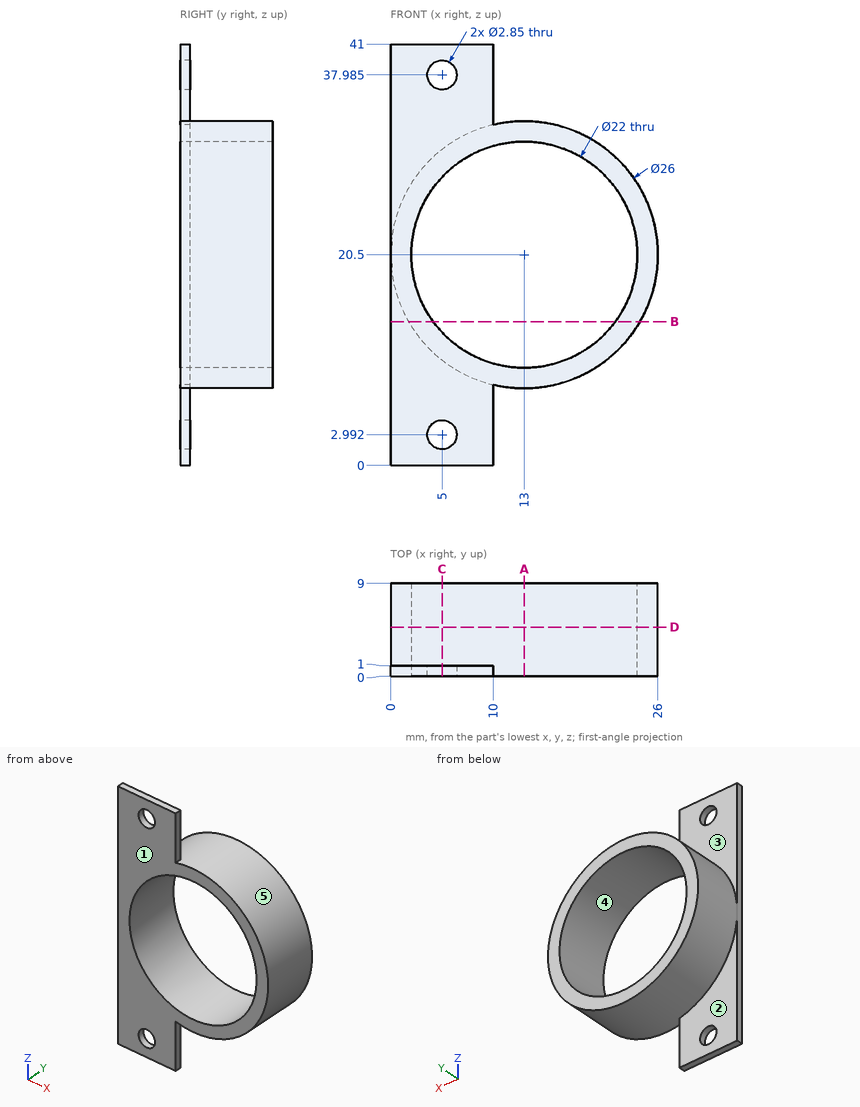
Design review of the part shown in the three views and the two pictorial views. Dimensions are in mm from the part's minimum x, y and z. A direction names the side the tool comes from. Round coordinates to 2 decimals unless told otherwise and drop trailing zeros. Write each loop counter-clockwise with the first axis right and the second up, starting at its lowest first coordinate (ties: lowest second). Pieces come first, ordered by that corner, then holes. Notation, with made-up numbers: M 18.25,38.5 L 76.25,38.5 A18 ccw 76.25,70.5 Z; hole C -21.75,-27 d4. An arc over 180 degrees is marked long. One line per item, written item: value. Start each with the question number.
1. Take a section at A-A on x = 13. State the section outline as (y, z) points.
2. Clearance check with flat-ended pins moving along their axes: P1, Ø1.1, axis at y = 0.5, z = 38, coming from the +X side; P2, Ø1, axis at y = 2, z = 10, coming from the -X side (1 decimal); P3, Ø4.5, axis at x = 5, z = 37.99, coming from the +Y side; P4, Ø13, axis at x = 13, z = 20.5, coming from the +Y side. State where each tip first meets the part, or that it passes through.
3. Take a section at B-B on z = 14. State the section outline as (x, y) points.
4. Take a section at D-D on y = 4.75. State the section outline as (x, z) points, then the cut area to 3 significant figures.
5. To check wall thickness, follow probe 1 along Z at (x, y) = (13, 3); probe 2 along X at (y, z) = (2.5, 20.5); probe 3 along Z at (x, y) = (3, 3) (1 decimal). State the ranges of each line that lie inside material, in increasing order. Write a range as from..to.
6. For the marked faces 1 and 2, list the 3-axis set-ups (+Z, -Z, +X, -X, +Y, -Y) from which the entire face can be reached by the end or side of a thin tool; tool diameter is ignored.
7. Draft analysis for pull direction Z (two halves, no side actions). For the marked faces 3, 4 and 5, state which applies: pulls with the +Z half, pulls with the -Z half, needs draft (parallel to the pull), parting line crosses it, or undercut.
8. Take a section at C-C on x = 5. State the section outline as (y, z) points.
Computed:
1. outline: M 0,7.5 L 9,7.5 L 9,9.5 L 0,9.5 Z; M 0,31.5 L 9,31.5 L 9,33.5 L 0,33.5 Z
2. P1: stops at x = 10
2. P2: stops at x = 4.7
2. P3: stops at y = 1
2. P4: passes through
3. outline: M 0,0 L 4.13,0 L 4.13,9 L 1.74,9 L 1.74,1 L 0,1 Z; M 21.87,0 L 24.26,0 L 24.26,9 L 21.87,9 Z
4. outline: C 13,20.5 d26; hole C 13,20.5 d22
4. area: 151 mm²
5. probe 1: z = 7.5..9.5, 31.5..33.5
5. probe 2: x = 0..2, 24..26
5. probe 3: z = 12.2..15.9, 25.1..28.8
6. face 1: +Z, -Z, +X, -X, -Y
6. face 2: -Z, -X, +Y
7. face 3: needs draft
7. face 4: undercut
7. face 5: parting line crosses it
8. outline: M 0,0 L 1,0 L 1,1.57 L 0,1.57 Z; M 0,4.42 L 1,4.42 L 1,10.25 L 9,10.25 L 9,12.95 L 0,12.95 Z; M 0,28.05 L 9,28.05 L 9,30.75 L 1,30.75 L 1,36.56 L 0,36.56 Z; M 0,39.41 L 1,39.41 L 1,41 L 0,41 Z
